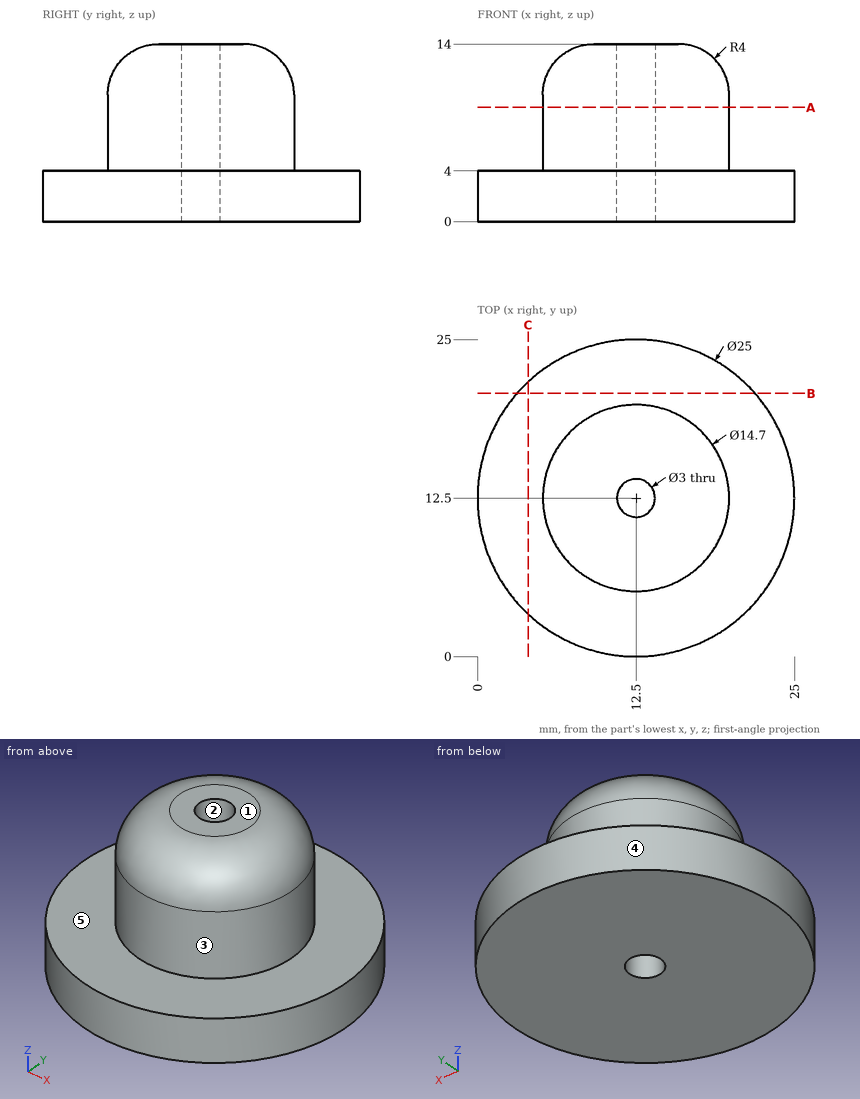
The drawing under review shows one solid part. Ordinate dimensions are in mm from its lowest x, y, z. A direction names the side the tool comes from. Round coordinates to 2 decimals unless told otherwise and drop trailing zeros. Write each loop counter-clockwise with the first axis right and the second up, starting at its lowest first coordinate (ties: lowest second). Pieces come first, ordered by that corner, then holes. Notation, with made-up numbers: (14.25, 27.25) - (60.25, 27.25) arc R22 cw to (60.25, 56.25) - close; hole circle Ø2 at (-24.75, -21). An arc over 180 degrees is marked (long way). Write each question's results on one line, items separated by ' | '.
Item 1: To check wall thickness, follow line 1 along Y through (x, z) = (12.5, 4.5); line 2 along Z through (x, y) = (2, 10.5); line 3 along Y through (x, z) = (13.5, 9.25). State the ranges of each line that lie inside material, in increasing order. Write a range as from..to.
Calculated:
line 1: y = 5.15..11, 14..19.85 | line 2: z = 0..4 | line 3: y = 5.22..11.38, 13.62..19.78
Item 2: Take a section at C-C on x = 4. State the section outline as (y, z) points, then the cut area to 3 significant figures.
Calculated:
outline: (3.33, 0) - (21.67, 0) - (21.67, 4) - (3.33, 4) - close | area: 73.3 mm^2
Item 3: Take a section at A-A on z = 9. State the section outline as (x, y) points.
Calculated:
outline: circle Ø14.7 at (12.5, 12.5); hole circle Ø3 at (12.5, 12.5)
Item 4: Draft analysis for pull direction X (two halves, no side actions). For the marked faces 1, 2 and 3, state which applies: pulls with the +X half, pulls with the -X half, needs draft (parallel to the pull), parting line crosses it, or undercut.
Calculated:
face 1: needs draft | face 2: undercut | face 3: parting line crosses it
Item 5: For pin 1 (1 mm diameter, centred on y = 9, z = 3, fed in from -X); pin 2 (3 mm diameter, centred on x = 8, z = 9, fed in from -Y); pin 3 (2.5 mm diameter, centred on x = 12.5, y = 12.5, fed in from -Z); pin 4 (1 mm diameter, centred on x = 16.5, z = 6.5, fed in from +Y), all flat-tipped, find the tip position at first contact; note any pin that passes through.
Calculated:
pin 1: stops at x = 0.37 | pin 2: stops at y = 5.79 | pin 3: passes through | pin 4: stops at y = 18.96
Item 6: Take a section at B-B on y = 20.75. State the section outline as (x, z) points, then the cut area to 3 significant figures.
Calculated:
outline: (3.11, 0) - (21.89, 0) - (21.89, 4) - (3.11, 4) - close | area: 75.1 mm^2
Item 7: For the marked faces 4 and 5, list the 3-axis set-ups (+Z, -Z, +X, -X, +Y, -Y) from which the entire face can be reached by the end or side of a thin tool; tool diameter is ignored.
Calculated:
face 4: +Z, -Z | face 5: +Z
